Geometry: final body of the model. Coordinates: model frame, mm. Coordinates: 2 decimals unless noted, no trailing zeros. Order: outer loops, then holes, each group sorted by start corner. A loop starts at its lowest first (then second) coordinate and runs counter-clockwise, first axis right, second up. Notation, with made-up numbers: M 60,-1 L 114,-1 A19 ccw 114,21 Z; hole C -36.75,-16.75 d9. An arc over 180 degrees is marked long. Write item = value, one per line. Start each with the question number.
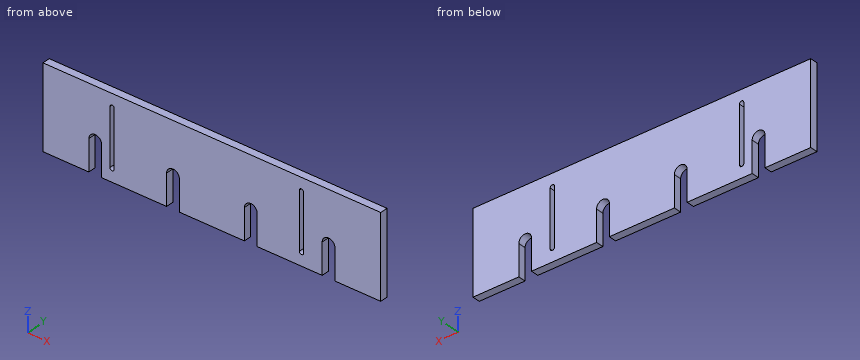
```python
from build123d import *

# Parameters (mm, degrees)
SKETCH50_W          = 419.1
SKETCH50_H          = 101.6
BOSS_EXTRUDE4_DEPTH = 9.525
CUT_EXTRUDE7_REACH  = 217.83
CUT_EXTRUDE8_REACH  = 217.83


with BuildPart() as part:
    # Sketch50 → Boss-Extrude4 (new body)
    with BuildSketch(Plane(origin=(0, 0, 0), x_dir=(1, 0, 0), z_dir=(0, 1, 0))):
        Rectangle(SKETCH50_W, SKETCH50_H)
    extrude(amount=BOSS_EXTRUDE4_DEPTH)

    # Sketch51 → Cut-Extrude7 (cut, up to next)
    with BuildSketch(Plane.XZ, mode=Mode.PRIVATE) as cut_extrude7_sk1:
        with BuildLine():
            Line((152.7175, -12.7), (152.7175, -50.8))
            ThreePointArc((152.7175, -50.8), (144.78, -58.7375), (136.8425, -50.8))
            Line((136.8425, -50.8), (136.8425, -12.7))
            ThreePointArc((136.8425, -12.7), (144.78, -4.7625), (152.7175, -12.7))
        make_face()
    cut_extrude7_tool1 = extrude(cut_extrude7_sk1.sketch, amount=-CUT_EXTRUDE7_REACH, mode=Mode.PRIVATE) & part.part
    # Sketch51 → Cut-Extrude7 (cut, up to next)
    with BuildSketch(Plane.XZ, mode=Mode.PRIVATE) as cut_extrude7_sk2:
        with BuildLine():
            Line((40.3225, -50.8), (40.3225, -12.7))
            ThreePointArc((40.3225, -12.7), (48.26, -4.7625), (56.1975, -12.7))
            Line((56.1975, -12.7), (56.1975, -50.8))
            ThreePointArc((56.1975, -50.8), (48.26, -58.7375), (40.3225, -50.8))
        make_face()
    cut_extrude7_tool2 = extrude(cut_extrude7_sk2.sketch, amount=-CUT_EXTRUDE7_REACH, mode=Mode.PRIVATE) & part.part
    cut_extrude7_1 = cut_extrude7_tool1.solids().sort_by_distance((144.78, 0, -31.75))[0]
    add(cut_extrude7_1, mode=Mode.SUBTRACT)
    cut_extrude7_2 = cut_extrude7_tool2.solids().sort_by_distance((48.26, 0, -31.75))[0]
    add(cut_extrude7_2, mode=Mode.SUBTRACT)
    cut_extrude7 = cut_extrude7_1 + cut_extrude7_2  # Cut-Extrude7 as one shape, for the pattern or mirror that repeats it

    # Mirror4: Cut-Extrude7 across plane
    add(cut_extrude7.mirror(Plane(origin=(0, 0, 0), x_dir=(0, 0, 1), z_dir=(1, 0, 0))), mode=Mode.SUBTRACT)

    # Sketch55 → Cut-Extrude8 (cut, up to next)
    with BuildSketch(Plane.XZ, mode=Mode.PRIVATE) as cut_extrude8_sk1:
        with BuildLine():
            Line((-126.492, 34.925), (-126.492, -34.925))
            ThreePointArc((-126.492, -34.925), (-123.825, -37.592), (-121.158, -34.925))
            Line((-121.158, -34.925), (-121.158, 34.925))
            ThreePointArc((-121.158, 34.925), (-123.825, 37.592), (-126.492, 34.925))
        make_face()
    cut_extrude8_tool1 = extrude(cut_extrude8_sk1.sketch, amount=-CUT_EXTRUDE8_REACH, mode=Mode.PRIVATE) & part.part
    # Sketch55 → Cut-Extrude8 (cut, up to next)
    with BuildSketch(Plane.XZ, mode=Mode.PRIVATE) as cut_extrude8_sk2:
        with BuildLine():
            Line((108.458, 34.925), (108.458, -34.925))
            ThreePointArc((108.458, -34.925), (111.125, -37.592), (113.792, -34.925))
            Line((113.792, -34.925), (113.792, 34.925))
            ThreePointArc((113.792, 34.925), (111.125, 37.592), (108.458, 34.925))
        make_face()
    cut_extrude8_tool2 = extrude(cut_extrude8_sk2.sketch, amount=-CUT_EXTRUDE8_REACH, mode=Mode.PRIVATE) & part.part
    add(cut_extrude8_tool1.solids().sort_by_distance((-123.825, 0, 0))[0], mode=Mode.SUBTRACT)
    add(cut_extrude8_tool2.solids().sort_by_distance((111.125, 0, 0))[0], mode=Mode.SUBTRACT)


solid = part.part
```
Item 1: Section query D-D on x = -44. Output: boundary loops of the cut face in (y, z) (3 decimals).
Item 2: Section query C-C on x = -144.78. Output: boundary loops of the cut face in (y, z) (1 decimal), and give its area (3 significant figures).
Item 3: Section query B-B on y = 8. Give the number of separate pieces and of enclosed holes in the cut face, and give its area (3 significant figures).
Item 4: Material intervals for probe 1 along X at (y, z) = (8.75, -42); probe 2 along X at (y, z) = (6, -2); probe 3 along Z at (x, y) = (-141, 3.25), sorted ascending. Write a range as [from, to].
Item 5: Section query A-A on z = 20. Output: boundary loops of the cut face in (x, y) (3 decimals).
Ans:
q1.outline = M 0,-6.003 L 9.525,-6.003 L 9.525,50.8 L 0,50.8 Z
q2.outline = M 0,-4.8 L 9.5,-4.8 L 9.5,50.8 L 0,50.8 Z
q2.area = 529 mm^2
q3.separate_pieces = 1
q3.enclosed_holes = 2
q3.area = 39,000 mm^2
q4.probe_1 = [-209.55, -152.72], [-136.84, -56.2], [-40.32, 40.32], [56.2, 136.84], [152.72, 209.55]
q4.probe_2 = [-209.55, -126.49], [-121.16, 108.46], [113.79, 209.55]
q4.probe_3 = [-5.72, 50.8]
q5.outline = M -209.55,0 L -126.492,0 L -126.492,9.525 L -209.55,9.525 Z; M -121.158,0 L 108.458,0 L 108.458,9.525 L -121.158,9.525 Z; M 113.792,0 L 209.55,0 L 209.55,9.525 L 113.792,9.525 Z
